Geometry: final body of the model. Coordinates: model frame, mm. Face numbers are marked on the shaded views. A direction names the side the tool comes from. Give positions to 0.01 mm unless a question says otherwise; leave off trailing zeros. Order: outer loops, then holes, each group sorted by start corner. A loop starts at its lowest first (then second) coordinate and runs counter-clockwise, first axis right, second up. Notation, with made-up numbers: (55, 5) -> (85, 5) arc R30 cw to (85, 33) -> close; hole circle Ø6 at (84.25, 51). An arc over 180 degrees is marked (long way). Answer in a Markdown table with one row per item. Add a question column.
Q1. Line query: line 1 along Y through (x, z) = (3, 0.2); line 2 along X through (y, z) = (-2, -0.05); line 3 along X through (y, z) = (-2, 0.4). Output: solid intervals per line, ascending. Write a range as from..to.
Q2. Contact query for flat-ended pins moving along their axis: P1, Ø0.8, axis at x = 2, z = 0.5, coming from the +Y side; P2, Ø0.5, axis at x = 5, z = 0.5, coming from the -Y side; P3, Ø0.8, axis at x = 4.5, y = 3, coming from the +Z side; P4, Ø0.8, axis at y = 0, z = 1, coming from the -X side. Output: stop coordinate, or through.
Q3. Pull-direction query (Y, two-part tool) for the marked faces 1, 2, 3 and 4; classes: +Y half, -Y half, draft (parallel to the pull), parting line (faces both ways), or undercut.
Q4. Set-up query: the marked faces 5 and 6. Return all of +Z, -Z, +X, -X, +Y, -Y with unobstructed straight access to the full face (end or side cutting, diameter ignored); none if empty.
Q5. Cut plane A-A on x = 3.75. Return the cut outline in (y, z).
from build123d import *

# Parameters (mm, degrees)
CROQUIS5_W                = 7
CROQUIS5_H                = 1
SALIENTE_EXTRUIR1_DEPTH   = 1
SALIENTE_EXTRUIR1_2_DEPTH = 1
SALIENTE_EXTRUIR1_3_DEPTH = 1
CROQUIS14_W               = 2.54
CROQUIS14_H               = 7.62
SALIENTE_EXTRUIR2_DEPTH   = 10
CROQUIS16_R               = 0.6
SALIENTE_EXTRUIR4_DEPTH   = 5


with BuildPart() as part:
    # Croquis5 → Saliente-Extruir1 (new body)
    with BuildSketch(Plane.XY):
        with Locations((3.511240097, -1.933057617)):
            Rectangle(CROQUIS5_W, CROQUIS5_H)
    extrude(amount=SALIENTE_EXTRUIR1_DEPTH)



with BuildPart() as body_2:
    # Croquis5 → Saliente-Extruir1 2 (new body)
    with BuildSketch(Plane.XY):
        with Locations((3.511240097, 0.606942383)):
            Rectangle(CROQUIS5_W, CROQUIS5_H)
    extrude(amount=SALIENTE_EXTRUIR1_2_DEPTH)


with BuildPart() as body_3:
    # Croquis5 → Saliente-Extruir1 3 (new body)
    with BuildSketch(Plane.XY):
        with Locations((3.511240097, 3.146942383)):
            Rectangle(CROQUIS5_W, CROQUIS5_H)
    extrude(amount=SALIENTE_EXTRUIR1_3_DEPTH)


with BuildPart() as part_1:
    add(part.part)

    add(body_2.part)  # Saliente-Extruir2 merges body 2

    add(body_3.part)  # Saliente-Extruir2 merges body 3
    # Croquis14 → Saliente-Extruir2 (add)
    with BuildSketch(Plane(origin=(7.011240097, 0, 0), x_dir=(0, 0, -1), z_dir=(1, 0, 0))):
        with Locations((-0.5, 0.606942383)):
            Rectangle(CROQUIS14_W, CROQUIS14_H)
    extrude(amount=SALIENTE_EXTRUIR2_DEPTH)

    # Croquis16 → Saliente-Extruir4 (add)
    with BuildSketch(Plane(origin=(17.011240097, 0, 0), x_dir=(0, 0, -1), z_dir=(1, 0, 0))):
        with Locations((-0.5, 0.606942383)):
            Circle(CROQUIS16_R)
        with Locations((-0.5, 1.816942383)):
            Circle(CROQUIS16_R)
        with Locations((-0.5, -0.603057617)):
            Circle(CROQUIS16_R)
    extrude(amount=SALIENTE_EXTRUIR4_DEPTH)


solid = part_1.part
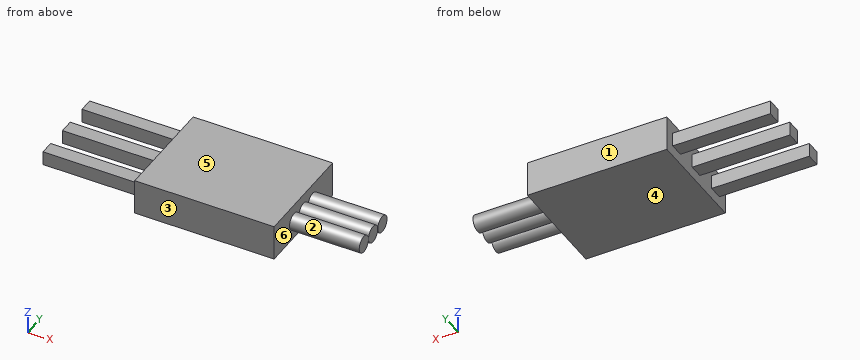
Completed:
| question | item | result |
|---|---|---|
| 1 | line 1 | y = -2.43..-1.43, 0.11..1.11, 2.65..3.65 |
| 1 | line 2 | x = 7.01..17.01 |
| 1 | line 3 | x = 0.01..17.01 |
| 2 | P1 | stops at y = 3.65 |
| 2 | P2 | stops at y = -2.43 |
| 2 | P3 | stops at z = 1 |
| 2 | P4 | stops at x = 0.01 |
| 3 | face 1 | +Y half |
| 3 | face 2 | undercut |
| 3 | face 3 | -Y half |
| 3 | face 4 | draft |
| 4 | face 5 | +Z, +X, -X, +Y, -Y |
| 4 | face 6 | +X |
| 5 | outline | (-2.43, 0) -> (-1.43, 0) -> (-1.43, 1) -> (-2.43, 1) -> close; (0.11, 0) -> (1.11, 0) -> (1.11, 1) -> (0.11, 1) -> close; (2.65, 0) -> (3.65, 0) -> (3.65, 1) -> (2.65, 1) -> close |
